Check sheet for the modelled part. Datum: model origin and axes. Units: mm. A direction names the side the tool comes from. Coordinates: 2 decimals unless noted, no trailing zeros. Order: outer loops, then holes, each group sorted by start corner. A loop starts at its lowest first (then second) coordinate and runs counter-clockwise, first axis right, second up.
1. Cross-section at A-A (y = -7). Enter the section's corners in (x, z), then the cut area to 3 significant figures.
2. Gauge pin test, flat ends, axial feed: pin 1 Ø4 at (x, z) = (7, 2.5) entering from -Y; pin 2 Ø3 at (y, z) = (-3.5, -0.5) entering from +X; pin 3 Ø6 at (x, y) = (-1.5, -8) entering from +Z; pin 4 Ø8 at (y, z) = (-7.5, 3) entering from -X. Record the tip position at first contact, or that the pin passes through.
3. Set-up check for faces 1 (the flat face through (-6, 7, 2)), 2 (the cylindrical face through (1.802, -10.846, 5.723)), 3 (the flat face through (0, -22, 0)): record each of +Z, -Z, +X, -X, +Y, -Y from which the full face is reachable in a straight line by a thin tool's end or side.
4. Thickness scan on line 1 (Y direction, x = 5, z = 4.5); line 2 (Z direction, x = 4.25, y = 1.5); line 3 (X direction, y = -3, z = 0.25). Record the ranges inside material, lowest first.
```python
from build123d import *

# Parameters (mm, degrees)
CROQUIS1_R              = 6
SALIENTE_EXTRUIR1_DEPTH = 22
REDONDEO2_R             = 1
CROQUIS3_W              = 6
CROQUIS3_H              = 4.5
REDONDEO3_R             = 0.5


with BuildPart() as part:
    # Croquis1 → Saliente-Extruir1 (new body)
    with BuildSketch(Plane(origin=(0, 0, 0), x_dir=(1, 0, 0), z_dir=(0, 1, 0))):
        with Locations(Location((0, 0, 0), (0, 0, 270))):
            Circle(CROQUIS1_R)
    extrude(amount=-SALIENTE_EXTRUIR1_DEPTH)

    # Croquis2 → Revolución1 (revolve)
    with BuildSketch(Plane(origin=(0, 0, 0), x_dir=(0, 0, -1), z_dir=(1, 0, 0))):
        with BuildLine():
            Line((0, 0), (9, 0))
            ThreePointArc((9, 0), (8.62079124, 3.579455266), (7.5, 7))
            Line((7.5, 7), (0, 7))
            Line((0, 7), (0, 0))
        make_face()
    revolve(axis=Axis((0, 0, 0), (0, 1, 0)))

    # Redondeo2
    redondeo2_edges = [part.edges().sort_by_distance(p)[0] for p in [
        (0, 7, 7.5),
    ]]
    fillet(redondeo2_edges, radius=REDONDEO2_R)

    # Croquis3 → Revolución2 (revolve)
    with BuildSketch(Plane(origin=(0, 0, 0), x_dir=(0, 0, -1), z_dir=(1, 0, 0))):
        with Locations((3, 9.25)):
            Rectangle(CROQUIS3_W, CROQUIS3_H)
    revolve(axis=Axis((0, 7, 0), (0, 1, 0)))

    # Redondeo3
    redondeo3_edges = [part.edges().sort_by_distance(p)[0] for p in [
        (0, 11.5, 6),
    ]]
    fillet(redondeo3_edges, radius=REDONDEO3_R)


solid = part.part
```
Data:
1. outline: circle Ø12 at (0, 0)
1. area: 113 mm2
2. pin 1: stops at y = -22
2. pin 2: stops at x = 6
2. pin 3: stops at z = 6
2. pin 4: stops at x = -6
3. face 1: +Y
3. face 2: -Y
3. face 3: +Z, -Z, +X, -X, -Y
4. line 1: y = 0 to 7
4. line 2: z = -7.86 to 7.86
4. line 3: x = -5.99 to 5.99
